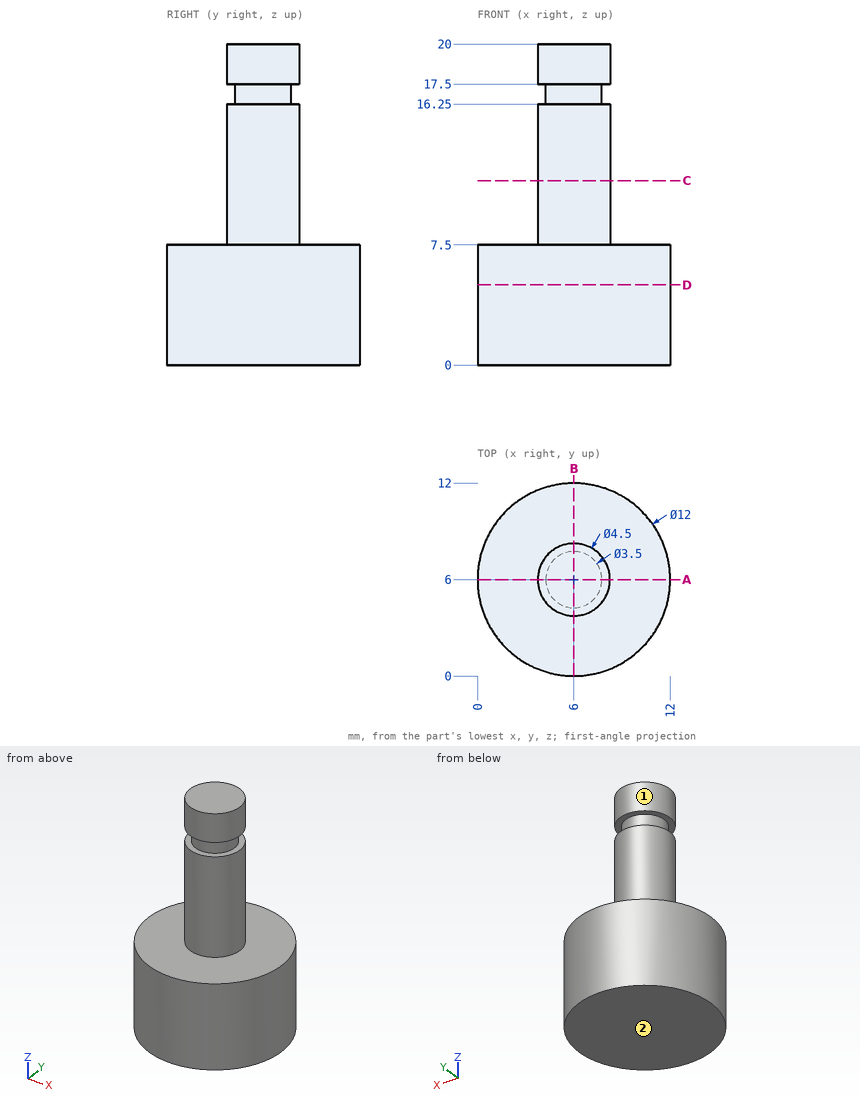
Source: three-view drawing plus pictorial views. Frame: mm from the lowest corner of the part. A direction names the side the tool comes from. Give positions to 0.01 mm unless a question says otherwise; leave off trailing zeros. Write each loop counter-clockwise with the first axis right and the second up, starting at its lowest first coordinate (ties: lowest second). Pieces come first, ordered by that corner, then holes. Notation, with made-up numbers: (42, 45.5) - (51, 45.5) arc R34 ccw to (51, 83.5) - close; hole circle Ø8 at (63.5, 88.25). An arc over 180 degrees is marked (long way). Write item = value, one per line. Start each with the question number.
Q1. Reachability of the marked faces 1 and 2 from +Z, -Z, +X, -X, +Y, -Y: full face, straight path, thin tool, end or side. Return the list, or none.
Q2. Cut plane D-D, the plane z = 5. Return loops of the section in (x, y).
Q3. Cut plane C-C, the plane z = 11.5. Return loops of the section in (x, y).
Q4. Cut plane A-A, the plane y = 6. Return loops of the section in (x, z).
Q5. Material intervals for probe 1 along Z at (x, y) = (8, 5.75); probe 2 along X at (y, z) = (6, 11.5); probe 3 along Z at (x, y) = (7.75, 10.5), sorted ascending.
Q6. Pin query (flat end, axial travel): pin 1 Ø2 at (x, y) = (2, 7.5) entering from +Z; pin 2 Ø4 at (y, z) = (10, 3.5) entering from +X; pin 3 Ø2 at (y, z) = (2.5, 12.5) entering from +X; pin 4 Ø2 at (x, z) = (7.5, 4.5) entering from -Y. Return the tip coordinate at first contact, or that it passes through.
Computed values:
q1.face_1 = +Z
q1.face_2 = -Z, +X, -X, +Y, -Y
q2.outline = circle Ø12 at (6, 6)
q3.outline = circle Ø4.5 at (6, 6)
q4.outline = (0, 0) - (12, 0) - (12, 7.5) - (8.25, 7.5) - (8.25, 16.25) - (7.75, 16.25) - (7.75, 17.5) - (8.25, 17.5) - (8.25, 20) - (3.75, 20) - (3.75, 17.5) - (4.25, 17.5) - (4.25, 16.25) - (3.75, 16.25) - (3.75, 7.5) - (0, 7.5) - close
q5.probe_1 = 0 to 16.25, 17.5 to 20
q5.probe_2 = 3.75 to 8.25
q5.probe_3 = 0 to 7.5
q6.pin_1 = 7.5
q6.pin_2 = 11.66
q6.pin_3 = through
q6.pin_4 = 0.02
